Source: three-view drawing plus pictorial views. Frame: mm from the lowest corner of the part. A direction names the side the tool comes from. Give positions to 0.01 mm unless a question says otherwise; leave off trailing zeros. Loops run counter-clockwise (first coordinate to the right, second up) from the corner with the lowest first, then second, coordinate; pieces in that order, holes last. Notation, with made-up numbers: (36.5, -20) - (69.5, -20) arc R29 cw to (69.5, 16) - close; hole circle Ø1 at (-36.75, -23.75). An arc over 180 degrees is marked (long way). Answer as a JSON object with one key per item and string values. Group by question number.
(1) Section query C-C (z = 3.5). Return loops of the section in (x, y), plus the area to 3 significant figures.
(2) Section query B-B (y = 15). Return loops of the section in (x, z), plus the area to 3 significant figures.
(3) Section query D-D (y = 24.75). Return loops of the section in (x, z).
(4) Pin query (flat end, axial travel): P1, Ø5, axis at y = 26.5, z = 19, coming from the +X side; P2, Ø4.5, axis at x = 14.5, z = 15, coming from the +Y side; P3, Ø16.5, axis at y = 16, z = 27, coming from the -X side; P4, Ø8, axis at x = 26.5, z = 6, coming from the -Y side. Return the tip coordinate at first contact, or that it passes through.
(5) Access query for the marked faces 1 and 2. Directions: +Z, -Z, +X, -X, +Y, -Y. A direction counts if a zero-diameter tool reaches every point of the face in a straight line with its end or side. Return the directions, or none.
(6) Section query A-A (x = 15). Return loops of the section in (y, z).
(7) Mould query, pull axis X, two halves, no side actions, for the marked faces 3, 4 and 5. Classes: +X half, -X half, draft (parallel to the pull), parting line (faces both ways), or undercut.
(8) Material intervals for L1, parallel to Y at x = 15, z = 8.35; L2, parallel to X at y = 20, z = 6.5; L3, parallel to X at y = 12.25, z = 23.5, sorted ascending.
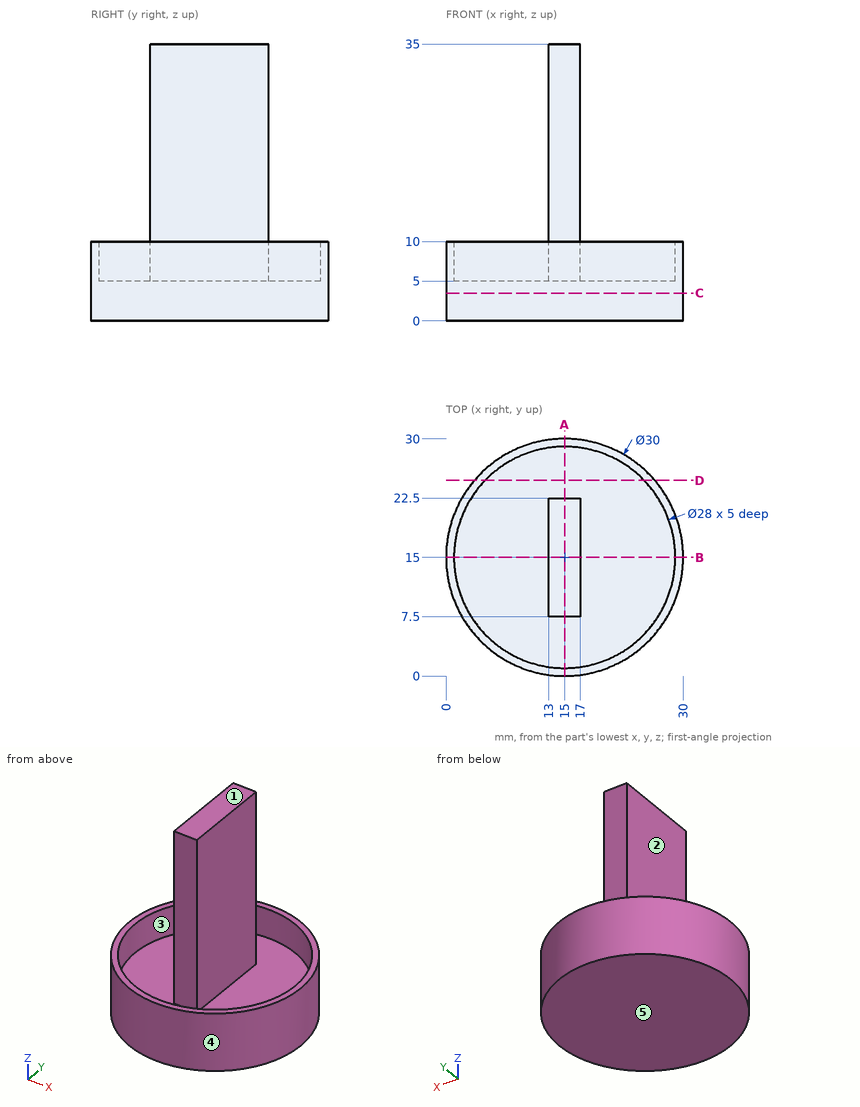
Recorded:
{
 "1": {"outline": "circle Ø30 at (15, 15)", "area": "707 mm^2"},
 "2": {"outline": "(0, 0) - (30, 0) - (30, 10) - (29, 10) - (29, 5) - (17, 5) - (17, 35) - (13, 35) - (13, 5) - (1, 5) - (1, 10) - (0, 10) - close", "area": "280 mm^2"},
 "3": {"outline": "(3.6, 0) - (26.4, 0) - (26.4, 10) - (25.05, 10) - (25.05, 5) - (4.95, 5) - (4.95, 10) - (3.6, 10) - close"},
 "4": {"P1": "passes through", "P2": "stops at y = 22.5", "P3": "stops at x = 13", "P4": "stops at y = 2.01"},
 "5": {"face 1": "+Z, +X, -X, +Y, -Y", "face 2": "+Z"},
 "6": {"outline": "(0, 0) - (30, 0) - (30, 10) - (29, 10) - (29, 5) - (22.5, 5) - (22.5, 35) - (7.5, 35) - (7.5, 5) - (1, 5) - (1, 10) - (0, 10) - close"},
 "7": {"face 3": "undercut", "face 4": "parting line", "face 5": "draft"},
 "8": {"L1": "y = 0 to 1, 7.5 to 22.5, 29 to 30", "L2": "x = 0.86 to 1.92, 13 to 17, 28.08 to 29.14", "L3": "x = 13 to 17"}
}
